Here's how the part is built. I have some questions about the finished solid (model axes, mm). Face numbers are marked on the shaded views. A direction names the side the tool comes from. Round coordinates to 2 decimals unless told otherwise and drop trailing zeros. Order: outer loops, then holes, each group sorted by start corner. A loop starts at its lowest first (then second) coordinate and runs counter-clockwise, first axis right, second up. Notation, with made-up numbers: (1.5, 0.25) -> (49.5, 0.25) arc R12 ccw to (49.5, 4.25) -> close; hole circle Ø8 at (13.25, -5). An arc over 180 degrees is marked (long way). Answer in a Markdown table with one row per item.
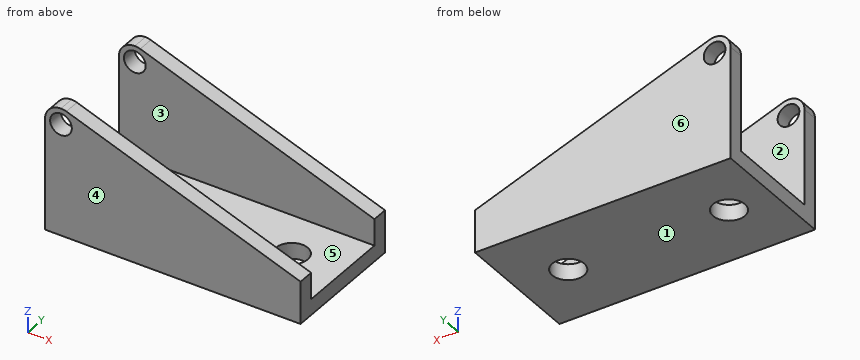
```python
from build123d import *

# Parameters (mm, degrees)
F0_R     = 2.159
F1_DEPTH = 25.4
F3_DEPTH = 50.801
F4_R     = 3.175
F5_DEPTH = 25.4


with BuildPart() as f1:
    # F0 (on Front) → F1 (new body)
    with BuildSketch(Plane.XZ):
        with BuildLine():
            ThreePointArc((-21.150258, 12.512567), (-21.679518, 12.652791), (-22.225, 12.7))
            ThreePointArc((-22.225, 12.7), (-24.470064, 11.770064), (-25.4, 9.525))
            Line((-25.4, 9.525), (-25.4, -12.7))
            Line((-25.4, -12.7), (25.4, -12.7))
            Line((25.4, -12.7), (25.4, -4.233333))
            Line((25.4, -4.233333), (-21.150258, 12.512567))
        make_face()
        with Locations((-22.225, 9.525)):
            Circle(F0_R, mode=Mode.SUBTRACT)
    extrude(amount=F1_DEPTH)

    # F2 (on face) → F3 (cut, through all)
    with BuildSketch(Plane(origin=(-25.4, 0, 0), x_dir=(0, -1, 0), z_dir=(-1, 0, 0))):
        Polygon((3.175, 15.972704), (3.175, -9.525), (22.225, -9.525), (22.225, 16.476365), align=None)
    extrude(amount=-F3_DEPTH, mode=Mode.SUBTRACT)

    # F4 (on face) → F5 (cut)
    with BuildSketch(Plane.XY.offset(-9.525)):
        with Locations((-16.687769, -12.7)):
            Circle(F4_R)
        with Locations((15.263206, -12.7)):
            Circle(F4_R)
    extrude(amount=-F5_DEPTH, mode=Mode.SUBTRACT)


solid = f1.part
```
1. Suppose I cut it at C-C on x = -16. Write out the boundary of the cut face in (y, z) (3 decimals).
Numbers:
| item | result |
|---|---|
| outline | (-25.4, -12.7) -> (-15.8, -12.7) -> (-15.8, -9.525) -> (-22.225, -9.525) -> (-22.225, 10.66) -> (-25.4, 10.66) -> close; (-9.6, -12.7) -> (0, -12.7) -> (0, 10.66) -> (-3.175, 10.66) -> (-3.175, -9.525) -> (-9.6, -9.525) -> close |
2. Suppose I cut it at D-D on x = 0.5. Write out the boundary of the cut face in (y, z) (3 decimals), then the cut area to 3 significant figures.
Numbers:
| item | result |
|---|---|
| outline | (-25.4, -12.7) -> (0, -12.7) -> (0, 4.724) -> (-3.175, 4.724) -> (-3.175, -9.525) -> (-22.225, -9.525) -> (-22.225, 4.724) -> (-25.4, 4.724) -> close |
| area | 171 mm2 |
3. We'd pull the mould along Y, two halves only. Please class the marked faces 1, 2, 3 and 4: released by +Y, released by -Y, zero draft, split by the parting line, or undercut.
Numbers:
| item | result |
|---|---|
| face 1 | zero draft |
| face 2 | undercut |
| face 3 | undercut |
| face 4 | released by -Y |
4. Please list where these lines run through material, in increasing order: line 1 along Y through (x, z) = (-22, 4.25) (3 decimals); line 2 along X through (y, z) = (-12.25, -10.5); line 3 along Z through (x, y) = (-4, -3.75) (3 decimals).
Numbers:
| item | result |
|---|---|
| line 1 | y = -25.4 to -22.225, -3.175 to 0 |
| line 2 | x = -25.4 to -19.83, -13.54 to 12.12, 18.41 to 25.4 |
| line 3 | z = -12.7 to -9.525 |
5. Suppose I cut it at B-B on z = -7.5. Write out the boundary of the cut face in (x, y) (3 decimals).
Numbers:
| item | result |
|---|---|
| outline | (-25.4, -25.4) -> (25.4, -25.4) -> (25.4, -22.225) -> (-25.4, -22.225) -> close; (-25.4, -3.175) -> (25.4, -3.175) -> (25.4, 0) -> (-25.4, 0) -> close |
6. Suppose I cut it at A-A on y = -12.7. Write out the boundary of the cut face in (x, z) (3 decimals), then the cut area to 3 significant figures.
Numbers:
| item | result |
|---|---|
| outline | (-25.4, -12.7) -> (-19.863, -12.7) -> (-19.863, -9.525) -> (-25.4, -9.525) -> close; (-13.513, -12.7) -> (12.088, -12.7) -> (12.088, -9.525) -> (-13.513, -9.525) -> close; (18.438, -12.7) -> (25.4, -12.7) -> (25.4, -9.525) -> (18.438, -9.525) -> close |
| area | 121 mm2 |
7. For pin 1 Ø2 at (x, y) = (-1, -3) entering from +Z; pin 2 Ø9.5 at (x, y) = (9, -16) entering from +Z (3 decimals), each with a flat end and sliding along its axis, tell me the tip position at first contact or that it passes through.
Numbers:
| item | result |
|---|---|
| pin 1 | stops at z = 5.62 |
| pin 2 | stops at z = -9.525 |
8. For the marked faces 5 and 6, which set-ups out of +Z, -Z, +X, -X, +Y, -Y let a thin tool reach every point of the face, with its end or its side?
Numbers:
| item | result |
|---|---|
| face 5 | +Z, +X, -X |
| face 6 | +Z, -Z, +X, -X, +Y |
